Part model, mm, in its own coordinate system. Give positions to 0.01 mm unless a question says otherwise; leave off trailing zeros. Write each loop counter-clockwise with the first axis right and the second up, starting at its lowest first coordinate (ties: lowest second). Pieces come first, ordered by that corner, then holes. Notation, with made-up numbers: M 41.25,4.5 L 64.25,4.5 A35 ccw 64.25,43.5 Z; hole C 87.5,-25.75 d3. An arc over 180 degrees is marked long. Use a Markdown table: item, result.
Autodesk Inventor part; units mm, degrees
ref_plane "YZ Plane" through (0, 0, 0) normal (1, 0, 0) x (0, 1, 0)
ref_plane "XZ Plane" through (0, 0, 0) normal (0, 1, 0) x (-1, 0, 0)
ref_plane "XY Plane" through (0, 0, 0) normal (0, 0, 1) x (1, 0, 0)
sketch "Sketch1" plane through (0, 0, 0) normal (0, 1, 0) x (-1, 0, 0)
  line L0 (-75, 25) -> (75, 25)
  line L1 (75, 25) -> (75, -25)
  line L2 (75, -25) -> (-75, -25)
  line L3 (-75, -25) -> (-75, 25)
  line L4 (-75, 25) -> (75, -25) construction
  line L5 (75, 25) -> (-75, -25) construction
  line L6 (-75, -25) -> (-35, -25)
  line L7 (-35, -25) -> (-35, 25)
  line L8 (-35, 25) -> (-75, 25)
  line L9 (-75, 25) -> (-75, -25)
  line L10 (-35, 25) -> (-35, 75)
  line L11 (-35, 75) -> (75, 75)
  line L12 (75, 75) -> (75, 25)
  line L13 (-35, 75) -> (25, 75)
  line L14 (25, 75) -> (75, 25)
  point P0 (0, 0)
  point P1 (-35, -25)
  dimension "d0" = 150
  dimension "d1" = 50
  dimension "d57" = 40
  dimension "d58" = 50
  dimension "d59" = 50
  dimension "d60" = 60
extrude "Extrusion1" add sketch "Sketch1" along normal blind 3 contours L10 L11 L14 L0 | L0 L1 L2 L7
sketch "Sketch6" plane through (0, 3, 0) normal (0, 1, 0) x (1, 0, 0)
  line L0 (35, 25) -> (-75, 25)
  line L1 (0, 25) -> (0, 8)
  circle A0 centre (0, 8) radius 5.25
  line L2 (0, 8) -> (-53.4, 8)
  circle A1 centre (-53.4, 8) radius 5
  circle A2 centre (0, 8) radius 8
  circle A3 centre (0, 16) radius 1.75
  circle A4 centre (-8, 8) radius 1.75
  circle A5 centre (0, 0) radius 1.75
  circle A6 centre (8, 8) radius 1.75
  circle A7 centre (-53.4, 8) radius 12
  line L3 (-53.4, -4) -> (-53.4, 20)
  circle A8 centre (-53.4, 20) radius 1.75
  circle A9 centre (-65.4, 8) radius 1.75
  circle A10 centre (-53.4, -4) radius 1.75
  circle A11 centre (-41.4, 8) radius 1.75
  point P0 (0, 0)
  point P1 (75, 25)
  dimension "d49" = 24
  dimension "d40" = 17
  dimension "d41" = 10.5
  dimension "d42" = 53.4
  dimension "d43" = 10
  dimension "d44" = 3.5
  dimension "d47" = 360
  dimension "d50" = 3.5
  dimension "d53" = 360
extrude "Extrusion6" cut sketch "Sketch6" against normal through all contours A3 A2 L1 | A11 A7 L2 | L2 A7 A11 | L1 A2 A3 | A2 A3 L1 | L1 A3 A2 | A4 L2 A2 | A2 L2 A4 | A0 L2 L1 | L1 L2 A0 | A6 A2 | A2 A6 | A2 A4 L2 | L2 A4 A2 | A5 A2 | A2 A5 | A7 A11 L2 | L2 A11 A7 | A8 L3 A7 | A7 A8 | A10 A7 | A7 L3 A10 | A1 L3 L2 | L2 L3 A1 | L3 A8 A7 | A7 A10 L3 | L3 A1 | A9 A7 | A7 A9
fillet "Fillet1" radius 20 5 edges at (35, 1.5, -25) (35, 1.5, 75) (-25, 1.5, 75) (-75, 1.5, 25) (-75, 1.5, -25)
properties part number "TopMount"
1. Two-plate mould, pull along Z, no slides. Class faces 1 (the cylindrical face through (-68.986, 1.521, -19.297)), 2 (the flat face through (-19, 0, 26)), 3 (the cylindrical face through (-54.79, 1.52, 5.06)): released by +Z, released by -Z, zero draft, split by the parting line, or undercut.
Findings below:
| item | result |
|---|---|
| face 1 | released by -Z |
| face 2 | zero draft |
| face 3 | undercut |
2. Drop a flat-ended pin along its axis: P1, Ø1.5, axis at x = -49.5, y = 2.5, coming from the +Z side. Give the stop position or say it passes through.
Findings below:
| item | result |
|---|---|
| P1 | z = 51.25 |
3. Cut at B-B, the plane z = 0. Give the cut face in (x, y).
Findings below:
| item | result |
|---|---|
| outline | M -75,0 L -1.75,0 L -1.75,3 L -75,3 Z; M 1.75,0 L 35,0 L 35,3 L 1.75,3 Z |
4. Cut at A-A, the plane x = -41.4. Give the cut face in (y, z).
Findings below:
| item | result |
|---|---|
| outline | M 0,-25 L 3,-25 L 3,-9.75 L 0,-9.75 Z; M 0,-6.25 L 3,-6.25 L 3,58.6 L 0,58.6 Z |
5. Cut at C-C, the plane y = 0.45. State how many separate pieces and enclosed holes the cut face has, then the cut area to 3 significant figures.
Findings below:
| item | result |
|---|---|
| separate pieces | 1 |
| enclosed holes | 10 |
| area | 9,230 mm2 |
6. Drill centre lines: L1, parallel to X at y = 2.2, z = 4; L2, parallel to Z at x = -8, y = 2.1; L3, parallel to Z at x = 16, y = 2. Where is each one in solid material? Low to high.
Findings below:
| item | result |
|---|---|
| L1 | -75 to -55.15, -51.65 to 35 |
| L2 | -25 to -9.75, -6.25 to 75 |
| L3 | -24.97 to 74.97 |
7. Cut at D-D, the plane x = 0. Give the cut face in (y, z).
Findings below:
| item | result |
|---|---|
| outline | M 0,-25 L 3,-25 L 3,-17.75 L 0,-17.75 Z; M 0,-14.25 L 3,-14.25 L 3,-13.25 L 0,-13.25 Z; M 0,-2.75 L 3,-2.75 L 3,-1.75 L 0,-1.75 Z; M 0,1.75 L 3,1.75 L 3,75 L 0,75 Z |
